```python
from build123d import *

# Parameters (mm, degrees)
F3_DEPTH = 36
F4_R     = 1.1
F5_DEPTH = 8
F6_R     = 1.1
F7_DEPTH = 21


with BuildPart() as f1:
    # F0 (on Front) → F1 (revolve)
    with BuildSketch(Plane.XZ):
        Polygon((-19, 0), (-11.1, 0), (-11.1, 10), (0, 10), (0, 21), (-3, 21), (-3, 38), (-5, 38), (-5, 40), (-19, 40), align=None)
    revolve(axis=Axis((0, 0, 15.5), (0, 0, 1)))

    # F2 (on face) → F3 (cut)
    with BuildSketch(Plane.XY.offset(40)):
        with BuildLine():
            Line((11.490485, 16.793786), (8.662058, 13.965359))
            ThreePointArc((8.662058, 13.965359), (8.662058, 8.662058), (13.965359, 8.662058))
            Line((13.965359, 8.662058), (16.793786, 11.490485))
            Line((16.793786, 11.490485), (11.490485, 16.793786))
        make_face()
        with BuildLine():
            Line((-16.793786, 11.490485), (-13.965359, 8.662058))
            ThreePointArc((-13.965359, 8.662058), (-8.662058, 8.662058), (-8.662058, 13.965359))
            Line((-8.662058, 13.965359), (-11.490485, 16.793786))
            Line((-11.490485, 16.793786), (-16.793786, 11.490485))
        make_face()
        with BuildLine():
            Line((-11.490485, -16.793786), (-8.662058, -13.965359))
            ThreePointArc((-8.662058, -13.965359), (-8.662058, -8.662058), (-13.965359, -8.662058))
            Line((-13.965359, -8.662058), (-16.793786, -11.490485))
            Line((-16.793786, -11.490485), (-11.490485, -16.793786))
        make_face()
        with BuildLine():
            Line((16.793786, -11.490485), (13.965359, -8.662058))
            ThreePointArc((13.965359, -8.662058), (8.662058, -8.662058), (8.662058, -13.965359))
            Line((8.662058, -13.965359), (11.490485, -16.793786))
            Line((11.490485, -16.793786), (16.793786, -11.490485))
        make_face()
    extrude(amount=-F3_DEPTH, mode=Mode.SUBTRACT)

    # F4 (on face) → F5 (cut)
    with BuildSketch(Plane.XY.offset(40)):
        with Locations((0, 8.980256)):
            Circle(F4_R)
        with Locations((8.980256, 0)):
            Circle(F4_R)
        with Locations((0, -8.980256)):
            Circle(F4_R)
        with Locations((-8.980256, 0)):
            Circle(F4_R)
    extrude(amount=-F5_DEPTH, mode=Mode.SUBTRACT)

    # F6 (on face) → F7 (cut)
    with BuildSketch(Plane(origin=(0, 0, 0), x_dir=(1, 0, 0), z_dir=(0, 0, -1))):
        with Locations((11.313708, 11.313708)):
            Circle(F6_R)
        with Locations((-11.313708, 11.313708)):
            Circle(F6_R)
        with Locations((-11.313708, -11.313708)):
            Circle(F6_R)
        with Locations((11.313708, -11.313708)):
            Circle(F6_R)
        with BuildLine():
            Line((-4.762, 12), (-4.762, 0))
            ThreePointArc((-4.762, 0), (0, -4.762), (4.762, 0))
            Line((4.762, 0), (4.762, 12))
            ThreePointArc((4.762, 12), (0, 16.762), (-4.762, 12))
        make_face()
    extrude(amount=-F7_DEPTH, mode=Mode.SUBTRACT)


solid = f1.part
```
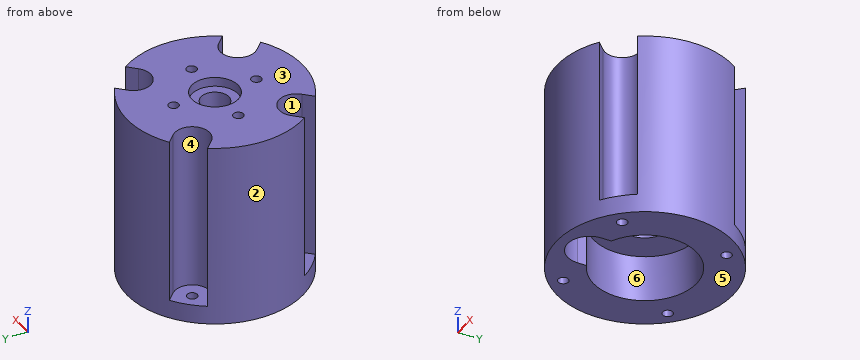
Source: CAD feature listing. Evaluate the final solid. Frame: model axes, mm. Face numbers are marked on the shaded views. A direction names the side the tool comes from. Coordinates: 2 decimals unless noted, no trailing zeros. Loops run counter-clockwise (first coordinate to the right, second up) from the corner with the lowest first, then second, coordinate; pieces in that order, holes last. Notation, with made-up numbers: M -6,-33 L 1,-33 A5 ccw 1,-25 Z; hole C 44.25,75 d1. An arc over 180 degrees is marked long. Use a Markdown table: item, result. Add a question column.
Q1. Access query for the marked faces 4, 5 and 6. Directions: +Z, -Z, +X, -X, +Y, -Y. A direction counts if a zero-diameter tool reaches every point of the face in a straight line with its end or side. Return the directions, or none.
Q2. Section query D-D, the plane y = -6. Return loops of the section in (x, z), and give its area (3 significant figures).
Q3. Draft query along Y for the marked faces 1, 2 and 3. Return one class per face: pulls with the +Y half, pulls with the -Y half, needs draft (parallel to the pull), parting line crosses it, or undercut.
Q4. Section query A-A, the plane x = 0. Return loops of the section in (y, z), and give its area (3 significant figures).
Q5. First-contact query: pin 1 (3.5 mm diameter, centred on x = 8.98, y = 0, fed in from -Z); pin 2 (1.5 mm diameter, centred on y = -0.5, z = 25, fed in from +X); pin 3 (6.5 mm diameter, centred on x = 13.5, y = -13, fed in from +Z); pin 4 (2 mm diameter, centred on x = 5, z = 10, fed in from +Y). Flat tips, straight axial feed; report the tip coordinate or a pass-through.
Q6. Section query C-C, the plane z = 34.5. Return loops of the section in (x, y), and give its area (3 significant figures).
Q7. Section query B-B, the plane z = 25. Return loops of the section in (x, y), and give its area (3 significant figures).
Q8. Material intervals for L1, parallel to Y at x = 0, z = 32.5; L2, parallel to Y at x = -9.5, z = 7.5; L3, parallel to Y at x = -8.5, z = 31, sorted ascending.
Result:
| question | item | result |
|---|---|---|
| 1 | face 4 | +Z |
| 1 | face 5 | -Z, +X, -X, +Y, -Y |
| 1 | face 6 | -Z |
| 2 | outline | M -18.03,0 L -9.34,0 L -9.34,10 L -4.76,10 L -4.76,21 L 4.76,21 L 4.76,10 L 9.34,10 L 9.34,0 L 18.03,0 L 18.03,40 L -18.03,40 Z |
| 2 | area | 1,150 mm2 |
| 3 | face 1 | undercut |
| 3 | face 2 | parting line crosses it |
| 3 | face 3 | needs draft |
| 4 | outline | M -19,0 L -16.76,0 L -16.76,21 L -3,21 L -3,38 L -5,38 L -5,40 L -7.88,40 L -7.88,32 L -10.08,32 L -10.08,40 L -19,40 Z; M 3,21 L 4.76,21 L 4.76,10 L 11.1,10 L 11.1,0 L 19,0 L 19,40 L 10.08,40 L 10.08,32 L 7.88,32 L 7.88,40 L 5,40 L 5,38 L 3,38 Z |
| 4 | area | 847 mm2 |
| 5 | pin 1 | stops at z = 10 |
| 5 | pin 2 | stops at x = 19 |
| 5 | pin 3 | stops at z = 4 |
| 5 | pin 4 | stops at y = 18.57 |
| 6 | outline | M -15.82,-10.52 L -13.97,-8.66 A3.75 cw -8.66,-13.97 L -10.52,-15.82 A19 ccw 10.52,-15.82 L 8.66,-13.97 A3.75 cw 13.97,-8.66 L 15.82,-10.52 A19 ccw 15.82,10.52 L 13.97,8.66 A3.75 cw 8.66,13.97 L 10.52,15.82 A19 ccw -10.52,15.82 L -8.66,13.97 A3.75 cw -13.97,8.66 L -15.82,10.52 A19 ccw Z; hole C -8.98,0 d2.2; hole C 0,0 d6; hole C 0,-8.98 d2.2; hole C 0,8.98 d2.2; hole C 8.98,0 d2.2 |
| 6 | area | 916 mm2 |
| 7 | outline | M -15.82,-10.52 L -13.97,-8.66 A3.75 cw -8.66,-13.97 L -10.52,-15.82 A19 ccw 10.52,-15.82 L 8.66,-13.97 A3.75 cw 13.97,-8.66 L 15.82,-10.52 A19 ccw 15.82,10.52 L 13.97,8.66 A3.75 cw 8.66,13.97 L 10.52,15.82 A19 ccw -10.52,15.82 L -8.66,13.97 A3.75 cw -13.97,8.66 L -15.82,10.52 A19 ccw Z; hole C 0,0 d6 |
| 7 | area | 931 mm2 |
| 8 | L1 | y = -19 to -10.08, -7.88 to -3, 3 to 7.88, 10.08 to 19 |
| 8 | L2 | y = -16.45 to -14.8, -8.03 to -5.74, 5.74 to 8.03, 14.8 to 16.45 |
| 8 | L3 | y = -16.99 to -13.79, -8.83 to 8.83, 13.79 to 16.99 |
